from build123d import *

# Parameters (mm, degrees)
SKETCH_1_R          = 3.5
EXTRUDE_1_DEPTH     = 4
SKETCH_2_R          = 3.5
EXTRUDE_2_DEPTH     = 10.9
SKETCH_3_W          = 4.5
SKETCH_3_H          = 4.5
EXTRUDE_3_DEPTH     = 2.5
SKETCH_6_R          = 3.25
CUT_EXTRUDE_1_DEPTH = 2.5


with BuildPart() as part:
    # 草图1 → 凸台-拉伸1 (new body)
    with BuildSketch(Plane(origin=(0, 0, 0), x_dir=(1, 0, 0), z_dir=(0, 1, 0))):
        Circle(SKETCH_1_R)
        with BuildLine():
            Line((-0.95, 1.2), (0.95, 1.2))
            ThreePointArc((0.95, 1.2), (1.376776695, 1.376776695), (1.2, 0.95))
            Line((1.2, 0.95), (1.2, -0.95))
            ThreePointArc((1.2, -0.95), (1.376776695, -1.376776695), (0.95, -1.2))
            Line((0.95, -1.2), (-0.95, -1.2))
            ThreePointArc((-0.95, -1.2), (-1.376776695, -1.376776695), (-1.2, -0.95))
            Line((-1.2, -0.95), (-1.2, 0.95))
            ThreePointArc((-1.2, 0.95), (-1.376776695, 1.376776695), (-0.95, 1.2))
        make_face(mode=Mode.SUBTRACT)
    extrude(amount=EXTRUDE_1_DEPTH)

    # 草图2 → 凸台-拉伸2 (add)
    with BuildSketch(Plane(origin=(0, 4, 0), x_dir=(1, 0, 0), z_dir=(0, 1, 0))):
        Circle(SKETCH_2_R)
    extrude(amount=EXTRUDE_2_DEPTH)

    # 草图3 → 凸台-拉伸3 (add)
    with BuildSketch(Plane(origin=(0, 14.9, 0), x_dir=(1, 0, 0), z_dir=(0, 1, 0))):
        Rectangle(SKETCH_3_W, SKETCH_3_H)
    extrude(amount=EXTRUDE_3_DEPTH)

    # 草图4 → 旋转1 (revolve)
    with BuildSketch(Plane(origin=(0, 17.4, 0), x_dir=(1, 0, 0), z_dir=(0, 1, 0))):
        with BuildLine():
            Line((0, 2.75), (0, 1.75))
            ThreePointArc((0, 1.75), (-0.5, 2.25), (0, 2.75))
        make_face()
        with BuildLine():
            Line((0, -1.75), (0, -2.75))
            ThreePointArc((0, -2.75), (-0.5, -2.25), (0, -1.75))
        make_face()
    revolve(axis=Axis((0, 17.4, -2.75), (0, 0, 1)))

    # 草图5 → 旋转2 (revolve)
    with BuildSketch(Plane(origin=(0, 17.4, 0), x_dir=(1, 0, 0), z_dir=(0, 1, 0))):
        with BuildLine():
            Line((-2.75, 0), (-1.75, 0))
            ThreePointArc((-1.75, 0), (-2.25, 0.5), (-2.75, 0))
        make_face()
        with BuildLine():
            Line((1.75, 0), (2.75, 0))
            ThreePointArc((2.75, 0), (2.25, 0.5), (1.75, 0))
        make_face()
    revolve(axis=Axis((-2.75, 17.4, 0), (1, 0, 0)))

    # 草图6 → 切除-拉伸1 (cut)
    with BuildSketch(Plane(origin=(0, 17.4, 0), x_dir=(1, 0, 0), z_dir=(0, 1, 0))):
        Circle(SKETCH_6_R)
    extrude(amount=CUT_EXTRUDE_1_DEPTH, mode=Mode.SUBTRACT)


solid = part.part
Here's how the part is built. I have some questions about the finished solid (model axes, mm). A direction names the side the tool comes from. Give positions to 0.01 mm unless a question says otherwise; leave off trailing zeros. Order: outer loops, then holes, each group sorted by start corner. A loop starts at its lowest first (then second) coordinate and runs counter-clockwise, first axis right, second up. Notation, with made-up numbers: M 7.5,70.5 L 60.5,70.5 A21 ccw 60.5,104.5 Z; hole C 1.25,-15.5 d11. An arc over 180 degrees is marked long. Answer as a JSON object with one key per item and string values. Group by question number.
1) Suppose I cut it at C-C, the plane x = 2.5. Write out the boundary of the cut face in (y, z).
2) Please list where these lines run through material, in increasing order: L1, parallel to Y at x = 1, z = 2.5; L2, parallel to Y at x = 0.5, z = 0.5; L3, parallel to X at y = 16, z = -1. Write a range as [from, to].
3) Suppose I cut it at D-D, the plane z = -0.25. Write out the boundary of the cut face in (x, y).
4) Suppose I cut it at B-B, the plane x = 0. Write out the boundary of the cut face in (y, z).
5) We'd pull the mould along Y, two halves only. Please class faces 3 (the flat face through (0, 0, 2)), 4 (the flat face through (0, 16, -2.25)), 5 (the flat face through (0, 2, -1.2)): pulls with the +Y half, pulls with the -Y half, needs draft (parallel to the pull), parting line crosses it, or undercut.
6) Suppose I cut it at A-A, the plane y = 3.75. Write out the boundary of the cut face in (x, z).
7) On a 3-axis mill with a long thin cutter (end or side, diameter ignored), from which of +Z, -Z, +X, -X, +Y, -Y can I reach the whole of each face in a straight line? I mean faces 1 (the flat face through (0, 4, 0)), 2 (the flat face through (0, 17.4, 0)). Say none if no direction works.
8) I'm going to push flat-ended pins straight in: pin 1 Ø2 at (y, z) = (5, -2) entering from +X; pin 2 Ø2 at (x, y) = (-0.5, 16.5) entering from -Z; pin 3 Ø1.2 at (y, z) = (16.5, 0) entering from -X. Where does each tip first touch, or does it pass through?
Results found:
{
 "1": {"outline": "M 0,-2.45 L 14.9,-2.45 L 14.9,2.45 L 0,2.45 Z; M 17.4,-0.43 L 17.4,0.43 A0.43 ccw Z"},
 "2": {"L1": "[0, 14.9]", "L2": "[4, 17.4]", "L3": "[-2.25, 2.25]"},
 "3": {"outline": "M -3.49,0 L -1.2,0 L -1.2,4 L 1.2,4 L 1.2,0 L 3.49,0 L 3.49,14.9 L 2.25,14.9 L 2.25,16.97 A0.43 ccw 2.68,17.4 L -2.68,17.4 A0.43 ccw -2.25,16.97 L -2.25,14.9 L -3.49,14.9 Z"},
 "4": {"outline": "M 0,-3.5 L 14.9,-3.5 L 14.9,-2.25 L 16.9,-2.25 A0.5 ccw 17.4,-2.75 L 17.4,2.75 A0.5 ccw 16.9,2.25 L 14.9,2.25 L 14.9,3.5 L 0,3.5 L 0,1.2 L 4,1.2 L 4,-1.2 L 0,-1.2 Z"},
 "5": {"face 3": "pulls with the -Y half", "face 4": "undercut", "face 5": "needs draft"},
 "6": {"outline": "C 0,0 d7; hole M -1.2,-0.95 A0.25 ccw long -0.95,-1.2 L 0.95,-1.2 A0.25 ccw long 1.2,-0.95 L 1.2,0.95 A0.25 ccw long 0.95,1.2 L -0.95,1.2 A0.25 ccw long -1.2,0.95 Z"},
 "7": {"face 1": "-Y", "face 2": "+Z, -Z, +X, -X, +Y"},
 "8": {"pin 1": "x = 3.35", "pin 2": "z = -2.75", "pin 3": "x = -2.65"}
}
